```python
from build123d import *

# Parameters (mm, degrees)
SKETCH1_R           = 3.9624
SKETCH1_R_2         = 1.5875
BOSS_EXTRUDE1_DEPTH = 0.3937
SKETCH5_W           = 0.58047107
SKETCH5_H           = 3.9624
CUT_EXTRUDE1_DEPTH  = 0.254


with BuildPart() as part:
    # Sketch1 → Boss-Extrude1 (new, symmetric)
    with BuildSketch(Plane(origin=(0, 0, 0), x_dir=(0, 0, -1), z_dir=(1, 0, 0))):
        Circle(SKETCH1_R)
        Circle(SKETCH1_R_2, mode=Mode.SUBTRACT)
    extrude(amount=BOSS_EXTRUDE1_DEPTH, both=True)

    # Sketch5 → Cut-Extrude1 (cut)
    with BuildSketch(Plane.ZY.offset(0.3937)):
        with Locations((0, 1.9812)):
            Rectangle(SKETCH5_W, SKETCH5_H)
    extrude(amount=-CUT_EXTRUDE1_DEPTH, mode=Mode.SUBTRACT)


solid = part.part
```
Verification items for the finished model (mm, model axes). Coordinates: 2 decimals unless noted, no trailing zeros. Order: outer loops, then holes, each group sorted by start corner. A loop starts at its lowest first (then second) coordinate and runs counter-clockwise, first axis right, second up. Notation, with made-up numbers: (59, -25.75) -> (63, -25.75) arc R27 ccw to (63, 7.25) -> close; hole circle Ø9 at (22.5, 16.25). An arc over 180 degrees is marked (long way). Answer as CSV lines item,"result". Start each with the question number.
1) Release check for a two-part mould opening along Z. For faces 1 (the face through (-0.394, -2, 0)), 2 (the face through (0.01, 3.93, 0.52)), 3 (the face through (-0.01, -1.55, 0.34)) record: released by +Z, released by -Z, zero draft, split by the parting line, or undercut.
2) Gauge pin test, flat end, axial feed: pin 1 Ø0.5 at (y, z) = (3, 0) entering from -X. Record the tip position at first contact, or that the pin passes through.
3) Cross-section at B-B, the plane z = 0. Record the boundary of the cut face in (x, y).
4) Cross-section at D-D, the plane z = 2.25. Record the boundary of the cut face in (x, y).
5) Cross-section at C-C, the plane x = 0. Record the boundary of the cut face in (y, z) (1 decimal), then the cut area to 3 significant figures.
6) Cross-section at A-A, the plane y = 0. Record the boundary of the cut face in (x, z), then the cut area to 3 significant figures.
7) Material ranges on L1, parallel to Z at x = 0.15, y = 0; L2, parallel to Z at x = -0.3, y = 3, recorded low to high. Write a range as [from, to].
Conclusion:
1,face 1,"zero draft"
1,face 2,"split by the parting line"
1,face 3,"undercut"
2,pin 1,"stops at x = -0.14"
3,outline,"(-0.39, -3.96) -> (0.39, -3.96) -> (0.39, -1.59) -> (-0.39, -1.59) -> close; (-0.14, 1.59) -> (0.39, 1.59) -> (0.39, 3.96) -> (-0.14, 3.96) -> close"
4,outline,"(-0.39, -3.26) -> (0.39, -3.26) -> (0.39, 3.26) -> (-0.39, 3.26) -> close"
5,outline,"circle Ø7.9 at (0, 0); hole circle Ø3.2 at (0, 0)"
5,area,"41.4 mm²"
6,outline,"(-0.39, -3.96) -> (0.39, -3.96) -> (0.39, -1.59) -> (-0.39, -1.59) -> close; (-0.39, 1.59) -> (0.39, 1.59) -> (0.39, 3.96) -> (-0.39, 3.96) -> close"
6,area,"3.74 mm²"
7,L1,"z = [-3.96, -1.59], [1.59, 3.96]"
7,L2,"z = [-2.59, -0.29], [0.29, 2.59]"
